Verification items for the finished model (mm, model axes). A direction names the side the tool comes from. Round coordinates to 2 decimals unless told otherwise and drop trailing zeros. Loops run counter-clockwise (first coordinate to the right, second up) from the corner with the lowest first, then second, coordinate; pieces in that order, holes last. Notation, with made-up numbers: (52, 60) - (62, 60) arc R9 ccw to (62, 71) - close; hole circle Ø5 at (87, 41). An arc over 180 degrees is marked (long way). Use CSV: the item, a comma, the result in double quotes.
```python
from build123d import *

# Parameters (mm, degrees)
BOSS_EXTRUDE1_DEPTH  = 40
BOSS_EXTRUDE2_DEPTH  = 5
FILLET1_R            = 5
CUT_EXTRUDE2_DEPTH   = 92.598097397
FILLET1_OF_MIRROR1_R = 5
SKETCH8_W            = 6
SKETCH8_H            = 3
CUT_EXTRUDE3_DEPTH   = 6


with BuildPart() as part:
    # Sketch1 → Boss-Extrude1 (new, symmetric)
    with BuildSketch(Plane.XY):
        with BuildLine():
            ThreePointArc((0.964181415, -1.149066665), (0.513030215, -1.409538931), (0, -1.5))
            Line((0, -1.5), (29.793839815, -1.5))
            ThreePointArc((29.793839815, -1.5), (28.733179643, -1.060660172), (28.293839815, 0))
            Line((28.293839815, 0), (28.293839815, 1.5))
            Line((28.293839815, 1.5), (4.121216129, 1.5))
            Line((4.121216129, 1.5), (0.964181415, -1.149066665))
        make_face()
        with BuildLine():
            Line((28.8296584, 26.149066665), (-0.964181415, 1.149066665))
            ThreePointArc((-0.964181415, 1.149066665), (-0.513030215, 1.409538931), (0, 1.5))
            Line((0, 1.5), (4.121216129, 1.5))
            Line((4.121216129, 1.5), (28.293839815, 21.783239619))
            Line((28.293839815, 21.783239619), (28.293839815, 25))
            ThreePointArc((28.293839815, 25), (28.434378134, 25.633927393), (28.8296584, 26.149066665))
        make_face()
        with BuildLine():
            Line((31.293839815, 0), (31.293839815, 25))
            ThreePointArc((31.293839815, 25), (31.153301495, 24.366072607), (30.758021229, 23.850933335))
            Line((30.758021229, 23.850933335), (28.293839815, 21.783239619))
            Line((28.293839815, 21.783239619), (28.293839815, 1.5))
            Line((28.293839815, 1.5), (29.793839815, 1.5))
            ThreePointArc((29.793839815, 1.5), (30.854499987, 1.060660172), (31.293839815, 0))
        make_face()
        with BuildLine():
            ThreePointArc((28.293839815, 0), (28.733179643, -1.060660172), (29.793839815, -1.5))
            ThreePointArc((29.793839815, -1.5), (30.854499987, -1.060660172), (31.293839815, 0))
            ThreePointArc((31.293839815, 0), (30.854499987, 1.060660172), (29.793839815, 1.5))
            Line((29.793839815, 1.5), (28.293839815, 1.5))
            Line((28.293839815, 1.5), (28.293839815, 0))
        make_face()
        with BuildLine():
            ThreePointArc((0, 1.5), (-0.513030215, 1.409538931), (-0.964181415, 1.149066665))
            ThreePointArc((-0.964181415, 1.149066665), (-1.409538931, -0.513030215), (0, -1.5))
            ThreePointArc((0, -1.5), (0.513030215, -1.409538931), (0.964181415, -1.149066665))
            Line((0.964181415, -1.149066665), (4.121216129, 1.5))
            Line((4.121216129, 1.5), (0, 1.5))
        make_face()
        with BuildLine():
            ThreePointArc((31.293839815, 25), (30.427767207, 26.359461681), (28.8296584, 26.149066665))
            ThreePointArc((28.8296584, 26.149066665), (28.434378134, 25.633927393), (28.293839815, 25))
            Line((28.293839815, 25), (28.293839815, 21.783239619))
            Line((28.293839815, 21.783239619), (30.758021229, 23.850933335))
            ThreePointArc((30.758021229, 23.850933335), (31.153301495, 24.366072607), (31.293839815, 25))
        make_face()
    extrude(amount=BOSS_EXTRUDE1_DEPTH, both=True)

    # Sketch5 → Boss-Extrude2 (add)
    with BuildSketch(Plane.XY.offset(40)):
        Polygon((-1.5, 0), (-1.5, 10), (31.293839815, 37.517298894), (31.293839815, 25), align=None)
    boss_extrude2 = extrude(amount=-BOSS_EXTRUDE2_DEPTH)

    # Fillet1
    fillet1_edges = [part.edges().sort_by_distance(p)[0] for p in [
        (-1.5, 10, 37.5),
        (31.293839815, 37.517298894, 37.5),
    ]]
    fillet(fillet1_edges, radius=FILLET1_R)

    # Sketch7 → Cut-Extrude2 (cut, symmetric)
    with BuildSketch(Plane.XY.offset(40)):
        with BuildLine():
            Line((1.852977001, 11.508074476), (7.981332546, 16.650375353))
            ThreePointArc((7.981332546, 16.650375353), (11.591201121, 16.334552776), (11.275378544, 12.724684201))
            Line((11.275378544, 12.724684201), (5.147022999, 7.582383323))
            ThreePointArc((5.147022999, 7.582383323), (1.537154424, 7.898205901), (1.852977001, 11.508074476))
        make_face()
        with BuildLine():
            Line((22.182635401, 28.566683341), (16.054279856, 23.424382464))
            ThreePointArc((16.054279856, 23.424382464), (15.738457279, 19.814513889), (19.348325854, 19.498691312))
            Line((19.348325854, 19.498691312), (25.476681399, 24.640992189))
            ThreePointArc((25.476681399, 24.640992189), (25.792503976, 28.250860764), (22.182635401, 28.566683341))
        make_face()
    cut_extrude2 = extrude(amount=CUT_EXTRUDE2_DEPTH, both=True, mode=Mode.SUBTRACT)

    # Mirror1: Boss-Extrude2, Cut-Extrude2 across plane
    add(boss_extrude2.mirror(Plane.XY))
    add(cut_extrude2.mirror(Plane.XY), mode=Mode.SUBTRACT)

    # Fillet1 of Mirror1
    fillet1_of_mirror1_edges = [part.edges().sort_by_distance(p)[0] for p in [
        (-1.5, 10, -37.5),
        (31.293839815, 37.517298894, -37.5),
    ]]
    fillet(fillet1_of_mirror1_edges, radius=FILLET1_OF_MIRROR1_R)

    # Sketch8 → Cut-Extrude3 (cut)
    with BuildSketch(Plane(origin=(31.293839815, 0, 0), x_dir=(0, 0, -1), z_dir=(1, 0, 0))):
        with Locations((0, 1.5)):
            Rectangle(SKETCH8_W, SKETCH8_H)
    extrude(amount=-CUT_EXTRUDE3_DEPTH, mode=Mode.SUBTRACT)


solid = part.part
```
1) Mould release check, pull along Y, two halves, no side actions. Record for faces 6 (the face through (-1.5, 4, 38)), 7 (the face through (4.87, 14.04, 37.47)), 8 (the face through (11.523, 20.928, 37.535)): +Y half, -Y half, draft (parallel to the pull), parting line (faces both ways), or undercut.
Returned:
face 6,"draft"
face 7,"undercut"
face 8,"+Y half"
2) Cross-section at D-D, the plane x = 13. Record the cut outline in (y, z).
Returned:
outline,"(-1.5, -40) - (1.5, -40) - (1.5, 40) - (-1.5, 40) - close; (8.95, -40) - (22.17, -40) - (22.17, -35) - (12.87, -35) - (12.87, 35) - (22.17, 35) - (22.17, 40) - (8.95, 40) - close"
3) Cross-section at B-B, the plane x = 21. Record the cut outline in (y, z), then the cut area to 3 significant figures.
Returned:
outline,"(-1.5, -40) - (1.5, -40) - (1.5, 40) - (-1.5, 40) - close; (15.66, -40) - (20.88, -40) - (20.88, -35) - (19.58, -35) - (19.58, 35) - (20.88, 35) - (20.88, 40) - (15.66, 40) - close; (27.57, -40) - (28.88, -40) - (28.88, -35) - (27.57, -35) - close; (27.57, 35) - (28.88, 35) - (28.88, 40) - (27.57, 40) - close"
area,"579 mm²"
4) Access from +Z, -Z, +X, -X, +Y, -Y to the whole of each face (thin tool, end or side, straight path). Record for faces 1 (the face through (28.48, 31.29, 37.47)), 2 (the face through (29, 1, -3)), 3 (the face through (11.523, 20.928, -37.535)), 4 (the face through (14.141, 13.824, 0.49)), 5 (the face through (19.16, 26.03, -37.53)).
Returned:
face 1,"+Z, -Z, +Y"
face 2,"+X"
face 3,"+Z, -Z, -X, +Y"
face 4,"-X, +Y"
face 5,"+Z, -Z"
5) Thickness scan on probe 1 along Z at (x, y) = (30, 27.5); probe 2 along Y at (x, z) = (16, -4); probe 3 along Y at (x, z) = (9, -4.5). Record the ranges inside material, lowest first. Write a range as [from, to].
Returned:
probe 1,"z = [-40, -35], [35, 40]"
probe 2,"y = [-1.5, 1.5], [11.47, 15.38]"
probe 3,"y = [-1.5, 1.5], [5.59, 9.51]"
6) Cross-section at C-C, the plane y = 20.5. Record the cut outline in (x, z).
Returned:
outline,"(11.01, -40) - (15.33, -40) - (15.33, -35) - (11.01, -35) - close; (11.01, 35) - (15.33, 35) - (15.33, 40) - (11.01, 40) - close; (20.54, -40) - (26.76, -40) - (26.76, 40) - (20.54, 40) - (20.54, 35) - (22.1, 35) - (22.1, -35) - (20.54, -35) - close; (28.29, -40) - (31.29, -40) - (31.29, 40) - (28.29, 40) - close"
7) Gauge pin test, flat ends, axial feed: pin 1 Ø6 at (y, z) = (13.5, -16.5) entering from -X; pin 2 Ø1.2 at (y, z) = (1, 1) entering from +X; pin 3 Ø1.5 at (x, z) = (17, 14) entering from +Y. Record the tip position at first contact, or that the pin passes through.
Returned:
pin 1,"stops at x = 10.18"
pin 2,"stops at x = 25.29"
pin 3,"stops at y = 16.85"
8) Cross-section at A-A, the plane z = -32. Record the cut outline in (x, y), then the cut area to 3 significant figures.
Returned:
outline,"(-0.96, 1.15) arc R1.5 ccw to (0, -1.5) - (29.79, -1.5) arc R1.5 ccw to (31.29, 0) - (31.29, 25) arc R1.5 ccw to (28.83, 26.15) - close; hole (4.12, 1.5) - (28.29, 1.5) - (28.29, 21.78) - close"
area,"275 mm²"
